Check sheet for the modelled part. Datum: model origin and axes. Units: mm. A direction names the side the tool comes from. Round coordinates to 2 decimals unless told otherwise and drop trailing zeros. Order: outer loops, then holes, each group sorted by start corner. A loop starts at its lowest first (then second) coordinate and runs counter-clockwise, first axis right, second up. Notation, with made-up numbers: (52.25, -29) -> (62.25, -29) arc R36 cw to (62.25, 9) -> close; hole circle Ø5 at (21.5, 38). An arc over 180 degrees is marked (long way). Answer in a Markdown table with one row per item.
```python
from build123d import *

# Parameters (mm, degrees)
F2_R    = 15
F3_SIZE = 2


with BuildPart() as f1:
    # F0 (on Front) → F1 (revolve)
    with BuildSketch(Plane.XZ):
        Polygon((24, 24.195369), (21, 24.195369), (21, 9.195369), (17, 0), (17, -15), (20, -15), (20, -0.62425), (24, 8.571119), align=None)
    revolve(axis=Axis((0, 0, 5.12058), (0, 0, -1)))

    # F2
    f2_edges = [f1.edges().sort_by_distance(p)[0] for p in [
        (-20, 0, -0.62425),
        (-24, 0, 8.571119),
        (-21, 0, 9.195369),
        (-17, 0, 0),
    ]]
    fillet(f2_edges, radius=F2_R)

    # F3
    f3_edges = [f1.edges().sort_by_distance(p)[0] for p in [
        (-21, 0, 24.195369),
        (-17, 0, -15),
    ]]
    chamfer(f3_edges, length=F3_SIZE)


solid = f1.part
```
(1) Scan lines: probe 1 along Y at (x, z) = (0, 14); probe 2 along Y at (x, z) = (0, -13). Record each from-to range of solid material in increasing order. Write a range as from..to.
Solutions:
| item | result |
|---|---|
| probe 1 | -24..-21, 21..24 |
| probe 2 | -20..-17, 17..20 |
(2) Section check B-B on z = -9. Record the boundary of the cut face in (x, y).
Solutions:
| item | result |
|---|---|
| outline | circle Ø40 at (0, 0); hole circle Ø34 at (0, 0) |
(3) Tool access check on faces 3 (the cylindrical face through (20.03, -6.31, 17.19)), 4 (the cylindrical face through (19.076, -6.007, -9.294)), 5 (the cylindrical face through (-23.977, -1.055, 18.031)). Record the directions out of +Z, -Z, +X, -X, +Y, -Y that give a thin tool (end or side, any length) a straight path to the whole face; none if there is none.
Solutions:
| item | result |
|---|---|
| face 3 | +Z |
| face 4 | -Z |
| face 5 | +Z, -Z |
(4) Draft check along Z on faces 1 (the flat face through (-18, 7, -15)), 2 (the conical face through (-4.58, 20.62, 22.32)). Enter one of: pulls with the +Z half, pulls with the -Z half, needs draft (parallel to the pull), parting line crosses it, or undercut.
Solutions:
| item | result |
|---|---|
| face 1 | pulls with the -Z half |
| face 2 | pulls with the +Z half |
(5) Section check A-A on z = 14. Record the boundary of the cut face in (x, y).
Solutions:
| item | result |
|---|---|
| outline | circle Ø48 at (0, 0); hole circle Ø42 at (0, 0) |
(6) Depth check by flat-ended pin: pin 1 Ø4 at (x, z) = (-5.5, 2) entering from -Y; pin 2 Ø1 at (y, z) = (-5.5, 1) entering from +X; pin 3 Ø2 at (x, z) = (-6.5, 17.5) entering from +Y. Enter the tip coordinate at first touch or a pass-through.
Solutions:
| item | result |
|---|---|
| pin 1 | y = -21.43 |
| pin 2 | x = 20.25 |
| pin 3 | y = 23.36 |
